Verification items for this drawing (mm, ordinates from the low corner). Round coordinates to 2 decimals unless told otherwise and drop trailing zeros. Order: outer loops, then holes, each group sorted by start corner. A loop starts at its lowest first (then second) coordinate and runs counter-clockwise, first axis right, second up. Notation, with made-up numbers: (39, -17.5) -> (49, -17.5) arc R23 ccw to (49, 1.5) -> close; hole circle Ø3 at (42, -31). An arc over 180 degrees is marked (long way). Return JSON: item names as keys, results as strings. Group by question number.
Item 1: Depth check by flat-ended pin: pin 1 Ø10 at (x, y) = (119, 110.475) entering from -Z; pin 2 Ø1 at (x, z) = (74.5, 3.5) entering from +Y. Enter the tip coordinate at first touch or a pass-through.
Item 2: Sectioned sample at B-B on y = 68.15. Record the cut outline in (x, z) (3 decimals).
Item 3: Sectioned sample at A-A on x = 91. Record the cut outline in (y, z).
Item 4: Sectioned sample at C-C on x = 44.5. Record the cut outline in (y, z), plus the area to 3 significant figures.
Item 5: Scan lines: probe 1 along Y at (x, z) = (91, 4.5); probe 2 along X at (y, z) = (33, 2.5); probe 3 along Y at (x, z) = (44.5, 1.5). Record each from-to range of solid material in increasing order. Write a range as from..to.
Item 6: Sectioned sample at D-D on z = 1. Give the number of separate pieces and of enclosed holes in the cut face, plus the area to 3 significant figures.
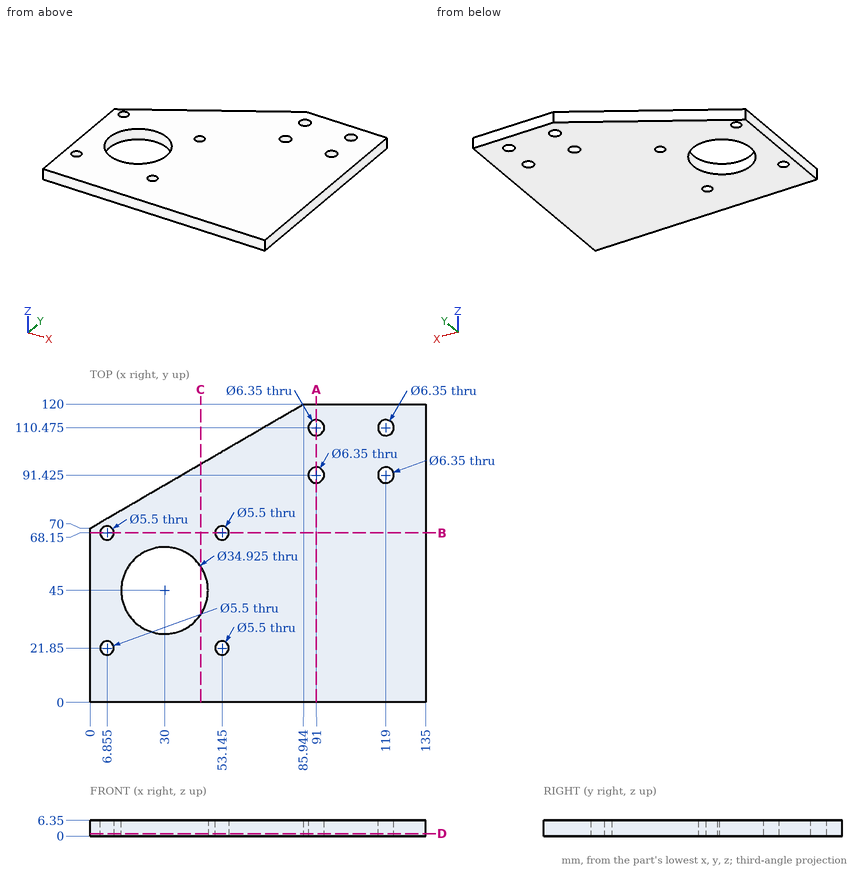
Recorded:
{
 "1": {"pin 1": "z = 0", "pin 2": "y = 113.63"},
 "2": {"outline": "(0, 0) -> (4.105, 0) -> (4.105, 6.35) -> (0, 6.35) -> close; (9.605, 0) -> (50.395, 0) -> (50.395, 6.35) -> (9.605, 6.35) -> close; (55.895, 0) -> (135, 0) -> (135, 6.35) -> (55.895, 6.35) -> close"},
 "3": {"outline": "(0, 0) -> (88.25, 0) -> (88.25, 6.35) -> (0, 6.35) -> close; (94.6, 0) -> (107.3, 0) -> (107.3, 6.35) -> (94.6, 6.35) -> close; (113.65, 0) -> (120, 0) -> (120, 6.35) -> (113.65, 6.35) -> close"},
 "4": {"outline": "(0, 0) -> (35.27, 0) -> (35.27, 6.35) -> (0, 6.35) -> close; (54.73, 0) -> (95.89, 0) -> (95.89, 6.35) -> (54.73, 6.35) -> close", "area": "485 mm²"},
 "5": {"probe 1": "0..88.25, 94.6..107.3, 113.65..120", "probe 2": "0..17.31, 42.69..135", "probe 3": "0..35.27, 54.73..95.89"},
 "6": {"separate pieces": "1", "enclosed holes": "9", "area": "12,900 mm²"}
}
